Can you work these out from the model? Positions are in its coordinate system, mm. Face numbers are marked on the shaded views. Round coordinates to 2 decimals unless told otherwise and drop trailing zeros. Write each loop counter-clockwise with the first axis right and the second up, starting at its lowest first coordinate (ties: lowest second). Pieces come first, ordered by that corner, then holes.
Q1. If we section it at A-A (z = 25): Please give me the cut outline in (x, y).
Q2. I'm going to push a flat-ended pin straight in: pin 1 Ø7 at (x, z) = (-11.1, 25) entering from +Y. Where does the tip first touch, or does it pass through?
Q3. We'd pull the mould along Z, two halves only. Please class the marked faces 1, 2 and 3: +Z half, -Z half, draft (parallel to the pull), parting line (faces both ways), or undercut.
Q4. Please list where these lines run through material, in increasing order: line 1 along Z through (x, y) = (-12, 2); line 2 along Z through (x, y) = (-9.5, -2.5); line 3 along Y through (x, z) = (-12, 34.5).
Q5. If we section it at B-B (y = 15): Please give me the cut outline in (x, z).
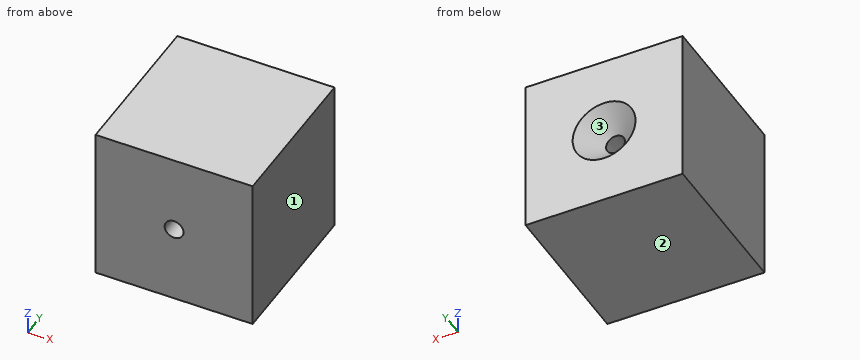
from build123d import *

# Parameters (mm, degrees)
SKETCH_1_W      = 50
SKETCH_1_H      = 50
EXTRUDE_1_DEPTH = 50


with BuildPart() as part:
    # 草图1 → 凸台-拉伸1 (new body)
    with BuildSketch(Plane.XY):
        with Locations((-11.096434238, -4.411764706)):
            Rectangle(SKETCH_1_W, SKETCH_1_H)
    extrude(amount=EXTRUDE_1_DEPTH)

    # 草图3 → 切除-旋转1 (revolve, cut)
    with BuildSketch(Plane(origin=(-11.096434238, 0, 0), x_dir=(0, 0, -1), z_dir=(1, 0, 0)), mode=Mode.PRIVATE) as cut_revolve_1_sk:
        Polygon((-25, 20.588235294), (-35, 20.588235294), (-28, 13.598319189), (-28, -29.411764706), (-25, -29.411764706), align=None)
    revolve(cut_revolve_1_sk.sketch.rotate(Axis((-11.096434238, 20.588235294, 25), (0, -1, 0)), 90), axis=Axis((-11.096434238, 20.588235294, 25), (0, -1, 0)), mode=Mode.SUBTRACT)


solid = part.part
A:
1. outline: (-36.1, -29.41) - (-14.1, -29.41) - (-14.1, 13.6) - (-21.1, 20.59) - (-36.1, 20.59) - close; (-8.1, -29.41) - (13.9, -29.41) - (13.9, 20.59) - (-1.1, 20.59) - (-8.1, 13.6) - close
2. pin 1: stops at y = 14.1
3. face 1: draft
3. face 2: -Z half
3. face 3: undercut
4. line 1: z = 0 to 22.14, 27.86 to 50
4. line 2: z = 0 to 22.46, 27.54 to 50
4. line 3: y = -29.41 to 20.13
5. outline: (-36.1, 0) - (13.9, 0) - (13.9, 50) - (-36.1, 50) - close; hole circle Ø8.81 at (-11.1, 25)
